```python
from build123d import *

# Parameters (mm, degrees)
SKETCH1_W               = 50.8
SKETCH1_H               = 25.4
BOSS_EXTRUDE1_DEPTH     = 9.525
CUT_EXTRUDE2_DEPTH      = 4.445
SKETCH2_R               = 2.2225
CUT_EXTRUDE1_DEPTH      = 9.525
CUT_EXTRUDE3_START      = -38.162422217
SKETCH5_R               = 2.2225
CUT_EXTRUDE3_DEPTH      = 41.337422217
MIRROR2_COPY_1_SKETCH_R = 2.2225
MIRROR2_COPY_1_DEPTH    = 9.525
FILLET1_R               = 1.5875


with BuildPart() as part:
    # Sketch1 → Boss-Extrude1 (new body)
    with BuildSketch(Plane.XY):
        Rectangle(SKETCH1_W, SKETCH1_H)
    extrude(amount=BOSS_EXTRUDE1_DEPTH)

    # Sketch4 → Cut-Extrude2 (cut, symmetric)
    with BuildSketch(Plane(origin=(0, 0, 0), x_dir=(1, 0, 0), z_dir=(0, 1, 0))):
        with BuildLine():
            Line((-16.22425, -6.6675), (-16.22425, -9.525))
            Line((-16.22425, -9.525), (-6.06425, -9.525))
            Line((-6.06425, -9.525), (-6.06425, -6.6675))
            ThreePointArc((-6.06425, -6.6675), (-11.14425, -1.5875), (-16.22425, -6.6675))
        make_face()
    cut_extrude2 = extrude(amount=CUT_EXTRUDE2_DEPTH, both=True, mode=Mode.SUBTRACT)

    # Sketch2 → Cut-Extrude1 (cut)
    with BuildSketch(Plane.XY.offset(9.525)):
        with Locations((-19.05, 7.9375)):
            Circle(SKETCH2_R)
    cut_extrude1 = extrude(amount=-CUT_EXTRUDE1_DEPTH, mode=Mode.SUBTRACT)

    # Sketch5 → Cut-Extrude3 (cut)
    with BuildSketch(Plane(origin=(0, 12.7, 0), x_dir=(1, 0, 0), z_dir=(0, 1, 0)).offset(CUT_EXTRUDE3_START)):
        with Locations(Location((-11.14425, -6.6675, 0), (0, 0, 180))):
            Circle(SKETCH5_R)
    cut_extrude3 = extrude(amount=CUT_EXTRUDE3_DEPTH, mode=Mode.SUBTRACT)

    # Mirror1: Cut-Extrude1 across plane
    add(cut_extrude1.mirror(Plane.ZX), mode=Mode.SUBTRACT)

    # Mirror2: Cut-Extrude2, Cut-Extrude1, Cut-Extrude3 across plane
    add(cut_extrude2.mirror(Plane.ZY), mode=Mode.SUBTRACT)
    add(cut_extrude1.mirror(Plane.ZY), mode=Mode.SUBTRACT)
    add(cut_extrude3.mirror(Plane.ZY), mode=Mode.SUBTRACT)

    # Mirror2 copy 1 sketch → Mirror2 copy 1 (cut)
    with BuildSketch(Plane(origin=(0, 0, 9.525), x_dir=(-1, 0, 0), z_dir=(0, 0, 1))):
        with Locations((-19.05, 7.9375)):
            Circle(MIRROR2_COPY_1_SKETCH_R)
    extrude(amount=-MIRROR2_COPY_1_DEPTH, mode=Mode.SUBTRACT)

    # Fillet1
    # the kernel refuses this fillet: 1.5875 mm, written as the material it takes off along each edge
    with BuildSketch(Plane(origin=(-23.8125, 11.1125, 7.9375), x_dir=(0, 1, 0), z_dir=(-1, 0, 0))) as fillet1_piece_1_section:
        Polygon((0, 0), (FILLET1_R, 0), (FILLET1_R, -FILLET1_R), (0, -FILLET1_R), align=None)
    fillet1_piece_1 = extrude(amount=FILLET1_R, mode=Mode.PRIVATE)
    fillet1_piece_1 = fillet1_piece_1 - Plane(origin=(-23.8125, 11.1125, 7.9375), x_dir=(0, -0.7071067811865475, -0.7071067811865475), z_dir=(-1, 0, 0)) * Sphere(FILLET1_R, mode=Mode.PRIVATE)
    add(fillet1_piece_1, mode=Mode.SUBTRACT)
    with BuildSketch(Plane(origin=(23.8125, 11.1125, 7.9375), x_dir=(0, 0, 1), z_dir=(0, 1, 0))) as fillet1_piece_2_section:
        Polygon((0, 0), (FILLET1_R, 0), (FILLET1_R, FILLET1_R), (0, FILLET1_R), align=None)
    fillet1_piece_2 = extrude(amount=FILLET1_R, mode=Mode.PRIVATE)
    fillet1_piece_2 = fillet1_piece_2 - Plane(origin=(23.8125, 11.1125, 7.9375), x_dir=(-0.7071067811865475, 0, -0.7071067811865475), z_dir=(0, 1, 0)) * Sphere(FILLET1_R, mode=Mode.PRIVATE)
    add(fillet1_piece_2, mode=Mode.SUBTRACT)
    with BuildSketch(Plane(origin=(-23.8125, -11.1125, 7.9375), x_dir=(0, -1, 0), z_dir=(-1, 0, 0))) as fillet1_piece_3_section:
        Polygon((0, 0), (FILLET1_R, 0), (FILLET1_R, FILLET1_R), (0, FILLET1_R), align=None)
    fillet1_piece_3 = extrude(amount=FILLET1_R, mode=Mode.PRIVATE)
    fillet1_piece_3 = fillet1_piece_3 - Plane(origin=(-23.8125, -11.1125, 7.9375), x_dir=(0, 0.7071067811865475, -0.7071067811865475), z_dir=(-1, 0, 0)) * Sphere(FILLET1_R, mode=Mode.PRIVATE)
    add(fillet1_piece_3, mode=Mode.SUBTRACT)
    with BuildSketch(Plane(origin=(23.8125, -11.1125, 7.9375), x_dir=(0, 0, 1), z_dir=(0, -1, 0))) as fillet1_piece_4_section:
        Polygon((0, 0), (FILLET1_R, 0), (FILLET1_R, -FILLET1_R), (0, -FILLET1_R), align=None)
    fillet1_piece_4 = extrude(amount=FILLET1_R, mode=Mode.PRIVATE)
    fillet1_piece_4 = fillet1_piece_4 - Plane(origin=(23.8125, -11.1125, 7.9375), x_dir=(-0.7071067811865475, 0, -0.7071067811865475), z_dir=(0, -1, 0)) * Sphere(FILLET1_R, mode=Mode.PRIVATE)
    add(fillet1_piece_4, mode=Mode.SUBTRACT)
    with BuildSketch(Plane(origin=(-23.8125, -11.1125, 1.5875), x_dir=(0, -1, 0), z_dir=(-1, 0, 0))) as fillet1_piece_5_section:
        Polygon((0, 0), (FILLET1_R, 0), (FILLET1_R, -FILLET1_R), (0, -FILLET1_R), align=None)
    fillet1_piece_5 = extrude(amount=FILLET1_R, mode=Mode.PRIVATE)
    fillet1_piece_5 = fillet1_piece_5 - Plane(origin=(-23.8125, -11.1125, 1.5875), x_dir=(0, 0.7071067811865475, 0.7071067811865475), z_dir=(-1, 0, 0)) * Sphere(FILLET1_R, mode=Mode.PRIVATE)
    add(fillet1_piece_5, mode=Mode.SUBTRACT)
    with BuildSketch(Plane(origin=(-23.8125, 11.1125, 1.5875), x_dir=(0, 1, 0), z_dir=(-1, 0, 0))) as fillet1_piece_6_section:
        Polygon((0, 0), (FILLET1_R, 0), (FILLET1_R, FILLET1_R), (0, FILLET1_R), align=None)
    fillet1_piece_6 = extrude(amount=FILLET1_R, mode=Mode.PRIVATE)
    fillet1_piece_6 = fillet1_piece_6 - Plane(origin=(-23.8125, 11.1125, 1.5875), x_dir=(0, -0.7071067811865475, 0.7071067811865475), z_dir=(-1, 0, 0)) * Sphere(FILLET1_R, mode=Mode.PRIVATE)
    add(fillet1_piece_6, mode=Mode.SUBTRACT)
    with BuildSketch(Plane(origin=(23.8125, 11.1125, 1.5875), x_dir=(0, 0, -1), z_dir=(0, 1, 0))) as fillet1_piece_7_section:
        Polygon((0, 0), (FILLET1_R, 0), (FILLET1_R, -FILLET1_R), (0, -FILLET1_R), align=None)
    fillet1_piece_7 = extrude(amount=FILLET1_R, mode=Mode.PRIVATE)
    fillet1_piece_7 = fillet1_piece_7 - Plane(origin=(23.8125, 11.1125, 1.5875), x_dir=(-0.7071067811865475, 0, 0.7071067811865475), z_dir=(0, 1, 0)) * Sphere(FILLET1_R, mode=Mode.PRIVATE)
    add(fillet1_piece_7, mode=Mode.SUBTRACT)
    with BuildSketch(Plane(origin=(23.8125, -11.1125, 1.5875), x_dir=(0, 0, -1), z_dir=(0, -1, 0))) as fillet1_piece_8_section:
        Polygon((0, 0), (FILLET1_R, 0), (FILLET1_R, FILLET1_R), (0, FILLET1_R), align=None)
    fillet1_piece_8 = extrude(amount=FILLET1_R, mode=Mode.PRIVATE)
    fillet1_piece_8 = fillet1_piece_8 - Plane(origin=(23.8125, -11.1125, 1.5875), x_dir=(-0.7071067811865475, 0, 0.7071067811865475), z_dir=(0, -1, 0)) * Sphere(FILLET1_R, mode=Mode.PRIVATE)
    add(fillet1_piece_8, mode=Mode.SUBTRACT)
    with BuildSketch(Plane(origin=(-23.8125, 12.7, 9.525), x_dir=(0, 0, -1), z_dir=(1, 0, 0)), Plane(origin=(23.8125, -12.7, 9.525), x_dir=(0, 0, -1), z_dir=(-1, 0, 0))) as fillet1_piece_9:
        with BuildLine():
            CenterArc((FILLET1_R, -FILLET1_R), FILLET1_R, 90, 90)
            Line((0, -FILLET1_R), (0, 0))
            Line((0, 0), (FILLET1_R, 0))
        make_face()
    extrude(amount=47.625, mode=Mode.SUBTRACT)
    with BuildSketch(Plane(origin=(-25.4, -11.1125, 9.525), x_dir=(0, 0, -1), z_dir=(0, 1, 0)), Plane(origin=(25.4, 11.1125, 0), x_dir=(-1, 0, 0), z_dir=(0, -1, 0))) as fillet1_piece_10:
        with BuildLine():
            CenterArc((FILLET1_R, -FILLET1_R), FILLET1_R, 90, 90)
            Line((0, -FILLET1_R), (0, 0))
            Line((0, 0), (FILLET1_R, 0))
        make_face()
    extrude(amount=22.225, mode=Mode.SUBTRACT)
    with BuildSketch(Plane(origin=(-25.4, -11.1125, 0), x_dir=(0, 0, 1), z_dir=(0, 1, 0)), Plane(origin=(25.4, 11.1125, 9.525), x_dir=(-1, 0, 0), z_dir=(0, -1, 0))) as fillet1_piece_11:
        with BuildLine():
            CenterArc((FILLET1_R, FILLET1_R), FILLET1_R, 180, 90)
            Line((0, FILLET1_R), (0, 0))
            Line((0, 0), (FILLET1_R, 0))
        make_face()
    extrude(amount=22.225, mode=Mode.SUBTRACT)
    with BuildSketch(Plane(origin=(-23.8125, 12.7, 0), x_dir=(0, 0, 1), z_dir=(1, 0, 0)), Plane(origin=(23.8125, -12.7, 0), x_dir=(0, 0, 1), z_dir=(-1, 0, 0))) as fillet1_piece_12:
        with BuildLine():
            CenterArc((FILLET1_R, FILLET1_R), FILLET1_R, 180, 90)
            Line((0, FILLET1_R), (0, 0))
            Line((0, 0), (FILLET1_R, 0))
        make_face()
    extrude(amount=47.625, mode=Mode.SUBTRACT)
    with BuildSketch(Plane(origin=(-25.4, -12.7, 1.5875), x_dir=(0, 1, 0), z_dir=(0, 0, 1)), Plane(origin=(25.4, -12.7, 1.5875), x_dir=(-1, 0, 0), z_dir=(0, 0, 1))) as fillet1_piece_13:
        with BuildLine():
            CenterArc((FILLET1_R, -FILLET1_R), FILLET1_R, 90, 90)
            Line((0, -FILLET1_R), (0, 0))
            Line((0, 0), (FILLET1_R, 0))
        make_face()
    extrude(amount=6.35, mode=Mode.SUBTRACT)
    with BuildSketch(Plane(origin=(-25.4, 12.7, 1.5875), x_dir=(0, -1, 0), z_dir=(0, 0, 1)), Plane(origin=(25.4, 12.7, 1.5875), x_dir=(-1, 0, 0), z_dir=(0, 0, 1))) as fillet1_piece_14:
        with BuildLine():
            CenterArc((FILLET1_R, FILLET1_R), FILLET1_R, 180, 90)
            Line((0, FILLET1_R), (0, 0))
            Line((0, 0), (FILLET1_R, 0))
        make_face()
    extrude(amount=6.35, mode=Mode.SUBTRACT)


solid = part.part
```
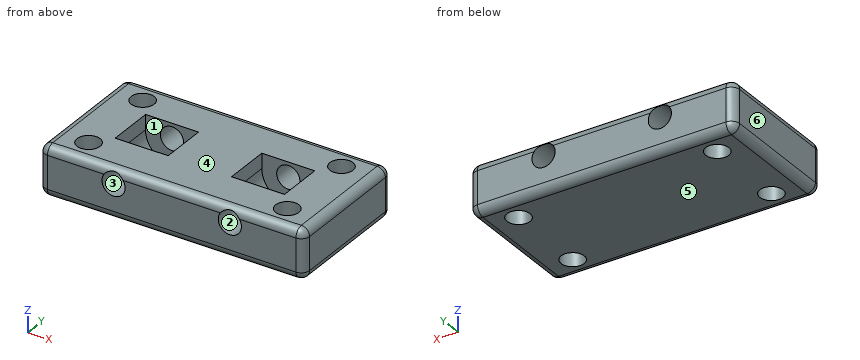
Read the model definition and answer for the solid it produces. Units are mm, in the model's axes. Face numbers are marked on the shaded views. A direction names the side the tool comes from. Round coordinates to 2 decimals unless told otherwise and drop trailing zeros. Write each loop counter-clockwise with the first axis right and the second up, starting at its lowest first coordinate (ties: lowest second). Pieces come first, ordered by that corner, then holes. Notation, with made-up numbers: (-23, -34.5) - (-13, -34.5) arc R15 cw to (-13, -24.5) - close; hole circle Ø5 at (0.25, 66.25). An arc over 180 degrees is marked (long way). One line per item, written item: value.
Q1. Find section B-B (y = -0.5). Determine the outline of the cut face in (x, z) (1 decimal).
The answers:
outline: (-25.4, 1.6) arc R1.6 ccw to (-23.8, 0) - (23.8, 0) arc R1.6 ccw to (25.4, 1.6) - (25.4, 7.9) arc R1.6 ccw to (23.8, 9.5) - (16.2, 9.5) - (16.2, 6.7) arc R5.1 cw to (6.1, 6.7) - (6.1, 9.5) - (-6.1, 9.5) - (-6.1, 6.7) arc R5.1 cw to (-16.2, 6.7) - (-16.2, 9.5) - (-23.8, 9.5) arc R1.6 ccw to (-25.4, 7.9) - close
Q2. For a pull along Z with two mould halves and no side action, classify the marked faces 3, 4, 5 and 6 as pulls with the +Z half, pulls with the -Z half, needs draft (parallel to the pull), parting line crosses it, or undercut.
The answers:
face 3: undercut
face 4: pulls with the +Z half
face 5: pulls with the -Z half
face 6: needs draft
Q3. Find section C-C (z = 5). Count the separate pieces of the cut face and the enclosed holes in it, and give its area (3 significant figures).
The answers:
separate pieces: 3
enclosed holes: 4
area: 958 mm2
Q4. Straight lines are drawn through the part: line 1 (Y direction, x = -11, z = 2.75) (3 decimals); line 2 (X direction, y = 4.25, z = 9); line 3 (X direction, y = -3.75, z = 5.5). For each, find the intervals that lie inside material, in ascending order. Write a range as from..to.
The answers:
line 1: y = -12.7..-4.445, 4.445..12.7
line 2: x = -24.99..-16.22, -6.06..6.06, 16.22..24.99
line 3: x = -25.4..-16.09, -6.2..6.2, 16.09..25.4
Q5. Find section A-A (x = -19.05). Determine the outline of the cut face in (y, z) (1 decimal).
The answers:
outline: (-12.7, 1.6) arc R1.6 ccw to (-11.1, 0) - (-10.2, 0) - (-10.2, 9.5) - (-11.1, 9.5) arc R1.6 ccw to (-12.7, 7.9) - close; (-5.7, 0) - (5.7, 0) - (5.7, 9.5) - (-5.7, 9.5) - close; (10.2, 0) - (11.1, 0) arc R1.6 ccw to (12.7, 1.6) - (12.7, 7.9) arc R1.6 ccw to (11.1, 9.5) - (10.2, 9.5) - close
Q6. Which of the six approach directions +Z, -Z, +X, -X, +Y, -Y give full straight-line access (tool end or side, diameter ignored) to the marked faces 1 and 2?
The answers:
face 1: +Z
face 2: +Y, -Y
Q7. Find section D-D (x = 12). Determine the outline of the cut face in (y, z) (1 decimal).
The answers:
outline: (-12.7, 1.6) arc R1.6 ccw to (-11.1, 0) - (11.1, 0) arc R1.6 ccw to (12.7, 1.6) - (12.7, 4.6) - (4.4, 4.6) - (4.4, 1.7) - (-4.4, 1.7) - (-4.4, 4.6) - (-12.7, 4.6) - close; (-12.5, 8.7) - (-4.4, 8.7) - (-4.4, 9.5) - (-11.1, 9.5) arc R1.6 ccw to start; (4.4, 8.7) - (12.5, 8.7) arc R1.6 ccw to (11.1, 9.5) - (4.4, 9.5) - close
